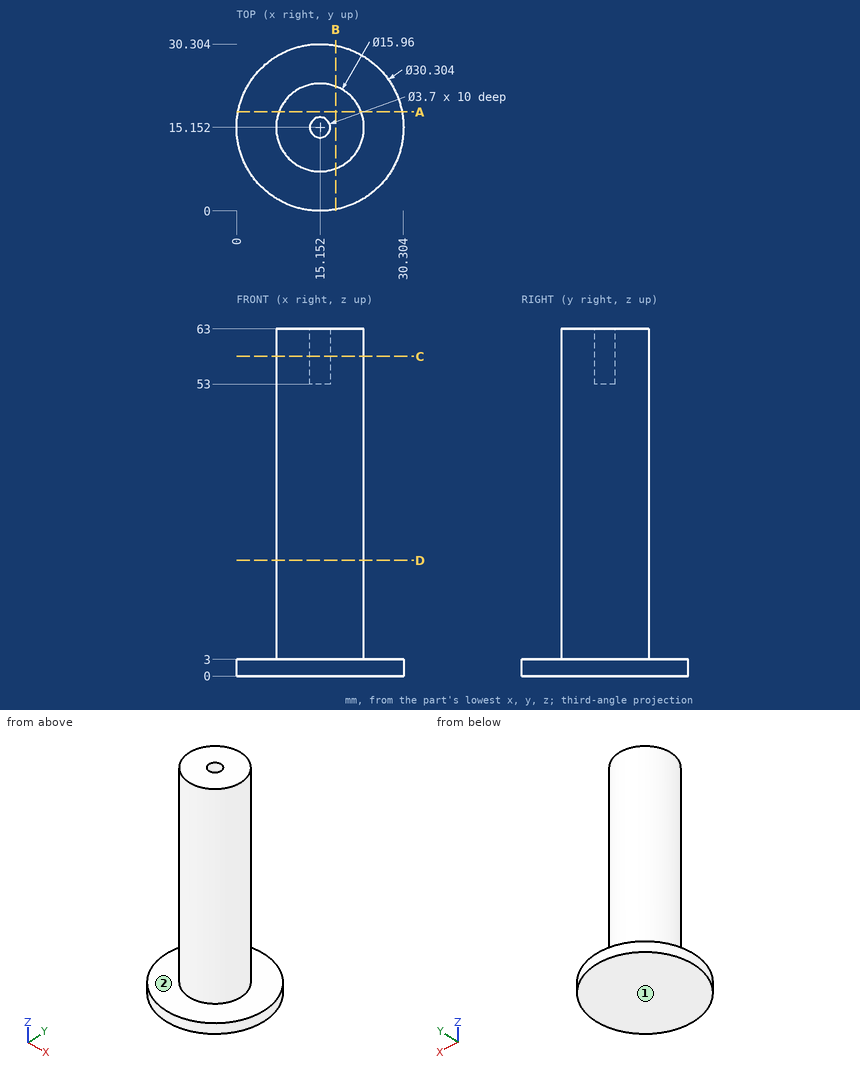
Answer from the drawing. Dimensions are ordinates in mm from the lowest x, y and z of the part. A direction names the side the tool comes from. Give positions to 0.01 mm unless a question says otherwise; leave off trailing zeros. Order: outer loops, then holes, each group sorted by start corner. A loop starts at its lowest first (then second) coordinate and runs counter-clockwise, first axis right, second up. Notation, with made-up numbers: (23.25, 15.5) -> (48.25, 15.5) arc R23 ccw to (48.25, 47.5) -> close; hole circle Ø9 at (85, 21). An arc over 180 degrees is marked (long way). Answer as a JSON object with one key per item and string values. Group by question number.
1. A tool of negligible diameter and unlimited length cuts with its end or side. For the marked faces 1 and 2, from which of +Z, -Z, +X, -X, +Y, -Y can it reach the whole face along a straight path? Write none if from no direction.
2. Flat-ended cylindrical pins translate along their axes: pin 1 Ø2 at (y, z) = (12.5, 21.5) entering from -X (1 decimal); pin 2 Ø12 at (y, z) = (9.5, 43) entering from +X; pin 3 Ø10 at (x, z) = (4.5, 20) entering from -Y; pin 4 Ø6 at (x, y) = (15.15, 15.15) entering from -Z. Find the tip coordinate at first contact, or state that the pin passes through.
3. Consider line 1 along X through (y, z) = (15, 19); line 2 along Z through (x, y) = (27, 14); line 3 along X through (y, z) = (18, 23.5). Determine where each line is inside the solid, lowest interval first. Write a range as [from, to].
4. Section C-C on z = 58 is taken. Determine the outline of the cut face in (x, y).
5. Section A-A on y = 18 is taken. Determine the outline of the cut face in (x, z) (1 decimal), plus the area to 3 significant figures.
6. Section D-D on z = 21 is taken. Determine the outline of the cut face in (x, y), plus the area to 3 significant figures.
Result sheet:
{
 "1": {"face 1": "-Z, +X, -X, +Y, -Y", "face 2": "+Z"},
 "2": {"pin 1": "stops at x = 7.3", "pin 2": "stops at x = 23.13", "pin 3": "stops at y = 9.52", "pin 4": "stops at z = 0"},
 "3": {"line 1": "x = [7.17, 23.13]", "line 2": "z = [0, 3]", "line 3": "x = [7.7, 22.61]"},
 "4": {"outline": "circle Ø15.96 at (15.15, 15.15); hole circle Ø3.7 at (15.15, 15.15)"},
 "5": {"outline": "(0.3, 0) -> (30, 0) -> (30, 3) -> (22.6, 3) -> (22.6, 63) -> (7.7, 63) -> (7.7, 3) -> (0.3, 3) -> close", "area": "984 mm^2"},
 "6": {"outline": "circle Ø15.96 at (15.15, 15.15)", "area": "200 mm^2"}
}
